Work out the finished part from the listing and answer in its coordinate system (mm). A direction names the side the tool comes from. Give positions to 0.01 mm unless a question says otherwise; leave off trailing zeros. Loops run counter-clockwise (first coordinate to the right, second up) from the corner with the lowest first, then second, coordinate; pieces in that order, holes last.
from build123d import *

# Parameters (mm, degrees)
PAD_DEPTH    = 35
SKETCH001_W  = 20
SKETCH001_H  = 15
PAD001_DEPTH = 2
FILLET_R     = 0.9
FILLET001_R  = 0.5
FILLET002_R  = 2
SKETCH002_W  = 16.059546
SKETCH002_H  = 5
PAD002_DEPTH = 10


with BuildPart() as part:
    # Sketch → Pad (new body)
    with BuildSketch(Plane.XY):
        with BuildLine():
            ThreePointArc((20, 0), (0, 6.835898), (-20, 0))
            Line((-20, -5.3), (-20, 0))
            Line((-5.65, -5.3), (-20, -5.3))
            Line((-5.65, -5.3), (-5.65, 0))
            Line((-5.65, 0), (5.65, 0))
            Line((5.65, 0), (5.65, -5.3))
            Line((20, -5.3), (5.65, -5.3))
            Line((20, 0), (20, -5.3))
        make_face()
        Polygon((-2.65, -5.3), (-5.65, -2.3), (-5.65, -5.3), align=None)
        Polygon((5.65, -5.3), (5.65, -2.3), (2.65, -5.3), align=None)
    extrude(amount=PAD_DEPTH)

    # Sketch001 (on Face13 of Pad) → Pad001 (join)
    with BuildSketch(Plane(origin=(0, 0, 0), x_dir=(1, 0, 0), z_dir=(0, 0, -1))):
        with Locations((0, -11.775117)):
            Rectangle(SKETCH001_W, SKETCH001_H)
    extrude(amount=-PAD001_DEPTH)

    # Fillet
    fillet_edges = [part.edges().sort_by_distance(p)[0] for p in [
        (0, 19.275117, 0),
        (0, 19.275117, 2),
    ]]
    fillet(fillet_edges, radius=FILLET_R)

    # Fillet001
    fillet001_edges = [part.edges().sort_by_distance(p)[0] for p in [
        (10, 19.275117, 1),
        (-10, 19.275117, 1),
    ]]
    fillet(fillet001_edges, radius=FILLET001_R)

    # Fillet002
    fillet002_edges = [part.edges().sort_by_distance(p)[0] for p in [
        (20, 0, 17.5),
        (-20, 0, 17.5),
    ]]
    fillet(fillet002_edges, radius=FILLET002_R)

    # Sketch002 (on Face24 of Fillet002) → Pad002 (join)
    with BuildSketch(Plane.XZ.offset(5.3)):
        with Locations((0, 2.5)):
            Rectangle(SKETCH002_W, SKETCH002_H)
    extrude(amount=-PAD002_DEPTH)


solid = part.part
Item 1: Find section A-A, the plane y = -1.5. Write down the section's boundary in (x, z), plus the area to 3 significant figures.
Item 2: Flat-ended cylindrical pins translate along their axes: pin 1 Ø12 at (y, z) = (3, 17.5) entering from +X; pin 2 Ø6 at (x, y) = (11.5, 14.5) entering from +Z; pin 3 Ø2.5 at (x, y) = (2.5, -2.5) entering from +Z; pin 4 Ø10 at (y, z) = (5.5, 24) entering from +X. Find the tip coordinate at first contact, or state that the pin passes through.
Item 3: Consider line 1 (X direction, y = -1, z = 30); line 2 (Z direction, x = -5, y = 16); line 3 (Z direction, x = -5, y = -1). Determine where each line is inside the solid, lowest interval first.
Item 4: For faces 4 (the face through (10, 12, 1)), 5 (the face through (20, -3, 17)), 6 (the face through (0, 0, 20)), determine the directions among +Z, -Z, +X, -X, +Y, -Y from which every point of the face is accessible in a straight line to the end or side of a thin tool.
Item 5: Find section C-C, the plane x = 6.5. Write down the section's boundary in (y, z).
Item 6: Determine the mould class of faces 1 (the face through (-10, 12, 1)), 2 (the face through (0, -3, 5)), 3 (the face through (0.287, 6.835, 17.255)) for opening direction X: released by +X, released by -X, zero draft, split by the parting line, or undercut.
Item 7: Find section B-B, the plane z = 21. Write down the section's boundary in (x, y).
Item 8: Find section D-D, the plane x = -4.5. Write down the section's boundary in (y, z).
Ans:
1. outline: (-20, 0) - (20, 0) - (20, 35) - (5.65, 35) - (5.65, 5) - (-5.65, 5) - (-5.65, 35) - (-20, 35) - close
1. area: 1,060 mm2
2. pin 1: stops at x = 20
2. pin 2: stops at z = 2
2. pin 3: stops at z = 5
2. pin 4: stops at x = 19.32
3. line 1: x = -20 to -5.65, 5.65 to 20
3. line 2: z = 0 to 2
3. line 3: z = 0 to 5
4. face 4: +Z, -Z, +X, +Y
4. face 5: +Z, -Z, +X, +Y, -Y
4. face 6: +Z
5. outline: (-5.3, 0) - (18.38, 0) arc R0.9 ccw to (19.28, 0.9) - (19.28, 1.1) arc R0.9 ccw to (18.38, 2) - (6.18, 2) - (6.18, 35) - (-5.3, 35) - close
6. face 1: released by -X
6. face 2: undercut
6. face 3: split by the parting line
7. outline: (-20, -5.3) - (-2.65, -5.3) - (-5.65, -2.3) - (-5.65, 0) - (5.65, 0) - (5.65, -2.3) - (2.65, -5.3) - (20, -5.3) - (20, -1) arc R2 ccw to (19.17, 0.62) arc R32.68 ccw to (-19.17, 0.62) arc R2 ccw to (-20, -1) - close
8. outline: (-5.3, 0) - (18.38, 0) arc R0.9 ccw to (19.28, 0.9) - (19.28, 1.1) arc R0.9 ccw to (18.38, 2) - (6.52, 2) - (6.52, 35) - (0, 35) - (0, 5) - (-3.45, 5) - (-3.45, 35) - (-5.3, 35) - close
